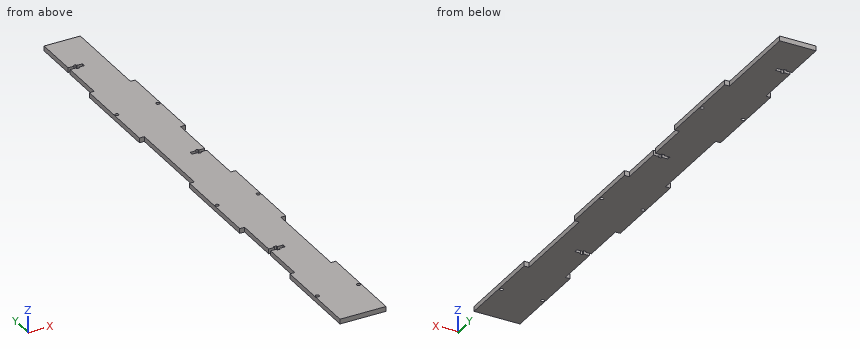
Autodesk Inventor part; units mm, degrees
ref_plane "YZ Plane" through (0, 0, 0) normal (1, 0, 0) x (0, 1, 0)
ref_plane "XZ Plane" through (0, 0, 0) normal (0, 1, 0) x (-1, 0, 0)
ref_plane "XY Plane" through (0, 0, 0) normal (0, 0, 1) x (1, 0, 0)
sketch "Sketch1" plane through (0, 0, 0) normal (0, 0, 1) x (1, 0, 0)
  line L0 (75.5009, -337.6029) -> (75.5009, -262.6029)
  line L1 (71.5009, -262.6029) -> (75.5009, -262.6029)
  line L2 (71.5009, -337.6029) -> (71.5009, -262.6029)
  line L3 (71.5009, -337.6029) -> (75.5009, -337.6029)
  line L4 (75.5009, -187.6029) -> (75.5009, -112.6029)
  line L5 (71.5009, -112.6029) -> (75.5009, -112.6029)
  line L6 (71.5009, -187.6029) -> (71.5009, -112.6029)
  line L7 (71.5009, -187.6029) -> (75.5009, -187.6029)
  line L8 (75.5009, -37.6029) -> (75.5009, 37.3971)
  line L9 (71.5009, 37.3971) -> (75.5009, 37.3971)
  line L10 (71.5009, -37.6029) -> (71.5009, 37.3971)
  line L11 (71.5009, -37.6029) -> (75.5009, -37.6029)
  line L12 (75.5009, 37.3971) -> (105.5009, 37.3971)
  line L13 (105.5009, 37.3971) -> (105.5009, -412.6029)
  line L14 (105.5009, -412.6029) -> (75.5009, -412.6029)
  line L15 (75.5009, -412.6029) -> (75.5009, 37.3971)
  line L16 (71.5009, -412.6029) -> (279.5009, -412.6029) construction
  line L17 (90.5009, -412.6029) -> (90.5009, 37.3971) construction
  line L18 (105.5009, -337.6029) -> (105.5009, -262.6029)
  line L19 (109.5009, -262.6029) -> (105.5009, -262.6029)
  line L20 (109.5009, -337.6029) -> (109.5009, -262.6029)
  line L21 (109.5009, -337.6029) -> (105.5009, -337.6029)
  line L22 (105.5009, -187.6029) -> (105.5009, -112.6029)
  line L23 (109.5009, -112.6029) -> (105.5009, -112.6029)
  line L24 (109.5009, -187.6029) -> (109.5009, -112.6029)
  line L25 (109.5009, -187.6029) -> (105.5009, -187.6029)
  line L26 (105.5009, -37.6029) -> (105.5009, 37.3971)
  line L27 (109.5009, 37.3971) -> (105.5009, 37.3971)
  line L28 (109.5009, -37.6029) -> (109.5009, 37.3971)
  line L29 (109.5009, -37.6029) -> (105.5009, -37.6029)
  line L30 (71.5009, -37.6029) -> (71.5009, -112.6029)
  line L31 (71.5009, -187.6029) -> (71.5009, -262.6029)
  line L32 (71.5009, -337.6029) -> (71.5009, -412.6029)
  line L33 (75.5009, -412.6029) -> (71.5009, -412.6029)
  line L34 (109.5009, -337.6029) -> (109.5009, -412.6029)
  line L35 (109.5009, -412.6029) -> (105.5009, -412.6029)
  line L36 (109.5009, -262.6029) -> (109.5009, -187.6029)
  line L37 (109.5009, -112.6029) -> (109.5009, -37.6029)
  line L38 (71.5009, -37.6029) -> (75.5009, -112.6029) construction
  circle A0 centre (73.5009, -75.1029) radius 1.5
  circle A1 centre (73.5009, -225.1029) radius 1.5
  circle A2 centre (73.5009, -375.1029) radius 1.5
  circle A3 centre (107.5009, -75.1029) radius 1.5
  circle A4 centre (107.5009, -225.1029) radius 1.5
  circle A5 centre (107.5009, -375.1029) radius 1.5
  line L39 (75.5009, -1.6029) -> (87.5009, -1.6029)
  line L40 (87.5009, -1.6029) -> (87.5009, 1.3971)
  line L41 (87.5009, 1.3971) -> (75.5009, 1.3971)
  line L42 (75.5009, 1.3971) -> (75.5009, -1.6029)
  line L43 (82.7009, 2.5971) -> (80.3009, 2.5971)
  line L44 (80.3009, 2.5971) -> (80.3009, -2.8029)
  line L45 (80.3009, -2.8029) -> (82.7009, -2.8029)
  line L46 (82.7009, -2.8029) -> (82.7009, 2.5971)
  line L47 (93.5009, -151.6029) -> (105.5009, -151.6029)
  line L48 (105.5009, -151.6029) -> (105.5009, -148.6029)
  line L49 (105.5009, -148.6029) -> (93.5009, -148.6029)
  line L50 (93.5009, -148.6029) -> (93.5009, -151.6029)
  line L51 (100.7009, -147.4029) -> (98.3009, -147.4029)
  line L52 (98.3009, -147.4029) -> (98.3009, -152.8029)
  line L53 (98.3009, -152.8029) -> (100.7009, -152.8029)
  line L54 (100.7009, -152.8029) -> (100.7009, -147.4029)
  line L55 (75.5009, -301.6029) -> (87.5009, -301.6029)
  line L56 (87.5009, -301.6029) -> (87.5009, -298.6029)
  line L57 (87.5009, -298.6029) -> (75.5009, -298.6029)
  line L58 (75.5009, -298.6029) -> (75.5009, -301.6029)
  line L59 (82.7009, -297.4029) -> (80.3009, -297.4029)
  line L60 (80.3009, -297.4029) -> (80.3009, -302.8029)
  line L61 (80.3009, -302.8029) -> (82.7009, -302.8029)
  line L62 (82.7009, -302.8029) -> (82.7009, -297.4029)
  point P0 (87.5009, -0.1029)
  point P1 (71.5009, -0.1029)
  point P2 (82.7009, -0.1029)
  point P3 (81.5009, 2.5971)
  point P4 (81.5009, -1.6029)
  point P5 (105.5009, -150.1029)
  point P6 (100.7009, -150.1029)
  point P7 (99.5009, -147.4029)
  point P8 (99.5009, -151.6029)
  point P9 (87.5009, -300.1029)
  point P10 (82.7009, -300.1029)
  point P11 (81.5009, -297.4029)
  point P12 (81.5009, -301.6029)
  point P13 (109.5009, -150.1029)
  point P14 (71.5009, -300.1029)
  point P15 (80.3009, 1.3971)
  point P16 (82.7009, 1.3971)
  point P17 (82.7009, -1.6029)
  point P18 (80.3009, -1.6029)
  point P19 (80.3009, -298.6029)
  point P20 (82.7009, -298.6029)
  point P21 (82.7009, -301.6029)
  point P22 (80.3009, -301.6029)
  point P23 (100.7009, -151.6029)
  point P24 (98.3009, -151.6029)
  point P25 (98.3009, -148.6029)
  point P26 (100.7009, -148.6029)
  dimension "d3" = 30
  dimension "d4" = 3
  dimension "d7" = 150
  dimension "d10" = 34
  dimension "d13" = 3
  dimension "d14" = 12
  dimension "d15" = 5.4
  dimension "d16" = 2.4
  dimension "d17" = 3
  dimension "d18" = 12
  dimension "d19" = 5.4
  dimension "d20" = 2.4
  dimension "d21" = 3
  dimension "d22" = 12
  dimension "d23" = 5.4
  dimension "d24" = 2.4
extrude "Extrusion1" add sketch "Sketch1" along normal blind 4 contours L15 L33 L32 L3 | L0 L55 L60 L61 L62 L56 L57 L59 L15 L4 L8 L39 L44 L45 L46 L40 L41 L43 L12 L13 L49 L54 L51 L52 L50 L47 L53 L14 | L31 L7 L15 L1 | L13 L21 L34 L35 | L30 L11 L15 L5 | L13 L25 L36 L19 | L23 L13 L29 L37
properties part number "Cableduct_Cover" material "MDF Medium Density Fiberboard"
Work out the finished part from the listing and answer in its coordinate system (mm). Give positions to 0.01 mm unless a question says otherwise; leave off trailing zeros. Loops run counter-clockwise (first coordinate to the right, second up) from the corner with the lowest first, then second, coordinate; pieces in that order, holes last. Notation, with made-up numbers: (-26.75, 18) -> (21.25, 18) arc R26 ccw to (21.25, 35) -> close; hole circle Ø9 at (3, 69). An arc over 180 degrees is marked (long way). Use CSV: the item, a comma, the result in double quotes.
1. The part is cut by section A-A (y = -120). Write down the section's boundary in (x, z), then the cut area to 3 significant figures.
Found:
outline,"(75.5, 0) -> (105.5, 0) -> (105.5, 4) -> (75.5, 4) -> close"
area,"120 mm^2"
2. The part is cut by section B-B (z = 1.2). State how many separate pieces and enclosed holes the cut face has, then the cut area to 3 significant figures.
Found:
separate pieces,"1"
enclosed holes,"6"
area,"15,100 mm^2"
3. Straight lines are drawn through the part: line 1 (Y direction, x = 108, z = 3.75); line 2 (Y direction, x = 84, z = 1.05); line 3 (Y direction, x = 82, z = 0.25). For each, find the intervals that lie inside material, in ascending order.
Found:
line 1,"-412.6 to -376.52, -373.69 to -337.6, -262.6 to -226.52, -223.69 to -187.6, -112.6 to -76.52, -73.69 to -37.6"
line 2,"-412.6 to -301.6, -298.6 to -1.6, 1.4 to 37.4"
line 3,"-412.6 to -302.8, -297.4 to -2.8, 2.6 to 37.4"
4. Flat-ended cylindrical pins translate along their axes: pin 1 Ø5 at (x, y) = (73.5, -375.1) entering from -Z; pin 2 Ø2 at (y, z) = (-169.5, 2) entering from +X; pin 3 Ø1.3 at (y, z) = (-152, 2.5) entering from -X. Find the tip coordinate at first contact, or state that the pin passes through.
Found:
pin 1,"z = 0"
pin 2,"x = 105.5"
pin 3,"x = 75.5"
